```python
from build123d import *

# Parameters (mm, degrees)
SKETCH1_W                        = 63.5
SKETCH1_H                        = 25.4
BOSS_EXTRUDE1_DEPTH              = 20.32
F_10_0_1935_DIAMETER_HOLE1_D     = 4.9149
F_10_0_1935_DIAMETER_HOLE1_DEPTH = 15.875
F_10_0_1935_DIAMETER_HOLE1_TIP   = 1.476584928
F_10_0_1935_DIAMETER_HOLE2_D     = 4.9149
F_10_0_1935_DIAMETER_HOLE2_DEPTH = 10.16
F_10_0_1935_DIAMETER_HOLE2_TIP   = 1.476584928
SKETCH6_R                        = 3.175
CUT_EXTRUDE1_DEPTH               = 59.427173695
SKETCH7_R                        = 7.62
CUT_EXTRUDE2_DEPTH               = 7.62
TAP_DRILL_FOR_M6X1_0_TAP1_D      = 5
TAP_DRILL_FOR_M6X1_0_TAP1_DEPTH  = 16.002
TAP_DRILL_FOR_M6X1_0_TAP1_TIP    = 1.502151548


with BuildPart() as part:
    # Sketch1 → Boss-Extrude1 (new body)
    with BuildSketch(Plane.XY):
        with Locations((-16.785267857, -8.961160714)):
            Rectangle(SKETCH1_W, SKETCH1_H)
    extrude(amount=BOSS_EXTRUDE1_DEPTH)

    # #10 (0.1935) Diameter Hole1
    with Locations(Plane(origin=(14.964732143, 0, 0), x_dir=(0, 0, -1), z_dir=(1, 0, 0))):
        with Locations((-10.16, -15.311160714)):
            Hole(F_10_0_1935_DIAMETER_HOLE1_D / 2, depth=F_10_0_1935_DIAMETER_HOLE1_DEPTH)
            with Locations((0, 0, -(F_10_0_1935_DIAMETER_HOLE1_DEPTH + F_10_0_1935_DIAMETER_HOLE1_TIP / 2))):  # 118° drill point
                Cone(0, F_10_0_1935_DIAMETER_HOLE1_D / 2, F_10_0_1935_DIAMETER_HOLE1_TIP, mode=Mode.SUBTRACT)

    # #10 (0.1935) Diameter Hole2
    with Locations(Plane.XY.offset(20.32)):
        with Locations((-0.910267857, -15.311160714)):
            Hole(F_10_0_1935_DIAMETER_HOLE2_D / 2, depth=F_10_0_1935_DIAMETER_HOLE2_DEPTH)
            with Locations((0, 0, -(F_10_0_1935_DIAMETER_HOLE2_DEPTH + F_10_0_1935_DIAMETER_HOLE2_TIP / 2))):  # 118° drill point
                Cone(0, F_10_0_1935_DIAMETER_HOLE2_D / 2, F_10_0_1935_DIAMETER_HOLE2_TIP, mode=Mode.SUBTRACT)

    # Sketch6 → Cut-Extrude1 (cut, through all)
    with BuildSketch(Plane(origin=(0, -21.661160714, 0), x_dir=(-1, 0, 0), z_dir=(0, -1, 0))):
        with Locations(Location((0.910267857, -10.16, 0), (0, 0, 90))):
            Circle(SKETCH6_R)
    extrude(amount=-CUT_EXTRUDE1_DEPTH, mode=Mode.SUBTRACT)

    # Sketch7 → Cut-Extrude2 (cut)
    with BuildSketch(Plane(origin=(0, 3.738839286, 0), x_dir=(1, 0, 0), z_dir=(0, 1, 0))):
        with Locations(Location((-0.910267857, -10.16, 0), (0, 0, 270))):
            Circle(SKETCH7_R)
    extrude(amount=-CUT_EXTRUDE2_DEPTH, mode=Mode.SUBTRACT)

    # Tap Drill for M6x1.0 Tap1
    with Locations(Plane(origin=(0, 3.738839286, 0), x_dir=(1, 0, 0), z_dir=(0, 1, 0))):
        with Locations((-43.455267857, -10.16)):
            Hole(TAP_DRILL_FOR_M6X1_0_TAP1_D / 2, depth=TAP_DRILL_FOR_M6X1_0_TAP1_DEPTH)
            with Locations((0, 0, -(TAP_DRILL_FOR_M6X1_0_TAP1_DEPTH + TAP_DRILL_FOR_M6X1_0_TAP1_TIP / 2))):  # 118° drill point
                Cone(0, TAP_DRILL_FOR_M6X1_0_TAP1_D / 2, TAP_DRILL_FOR_M6X1_0_TAP1_TIP, mode=Mode.SUBTRACT)


solid = part.part
```
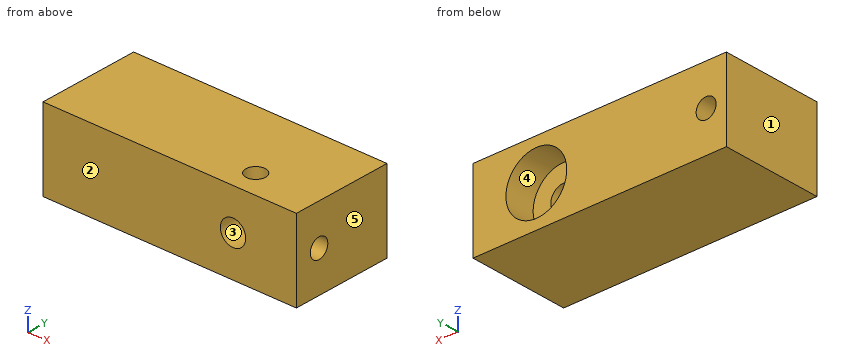
Check sheet for the modelled part. Datum: model origin and axes. Units: mm. Face numbers are marked on the shaded views. A direction names the side the tool comes from. Coordinates: 2 decimals unless noted, no trailing zeros. Loops run counter-clockwise (first coordinate to the right, second up) from the corner with the lowest first, then second, coordinate; pieces in that order, holes last.
1) Sectioned sample at C-C (y = -9). Record the boundary of the cut face in (x, z) (3 decimals).
2) Material ranges on probe 1 along X at (y, z) = (-9.25, 10); probe 2 along Y at (x, z) = (5, 10.25); probe 3 along X at (y, z) = (-6, 8.75) (3 decimals), recorded low to high.
3) Gauge pin test, flat ends, axial feed: pin 1 (4 mm diameter, centred on x = -0.91, y = -15.31, fed in from +Z); pin 2 (7.5 mm diameter, centred on x = -0.91, z = 10.16, fed in from +Y). Record the tip position at first contact, or that the pin passes through.
4) Release check for a two-part mould opening along X. For the marked faces 1, 2 and 3 record: released by +X, released by -X, zero draft, split by the parting line, or undercut.
5) Sectioned sample at D-D (y = 0.25). Record the boundary of the cut face in (x, z).
6) Sectioned sample at A-A (z = 16.25). Record the boundary of the cut face in (x, y).
7) Sectioned sample at B-B (x = 4). Record the boundary of the cut face in (y, z), and give its area (3 significant figures).
8) Access from +Z, -Z, +X, -X, +Y, -Y to the whole of each face (thin tool, end or side, straight path). Record for the marked faces 4 and 5.
Check sheet entries:
1. outline: (-48.535, 0) - (14.965, 0) - (14.965, 20.32) - (-48.535, 20.32) - close; hole circle Ø5 at (-43.455, 10.16); hole circle Ø6.35 at (-0.91, 10.16)
2. probe 1: x = -48.54 to -45.95, -40.96 to -4.08, 2.26 to 14.96
2. probe 2: y = -21.66 to -17.77, -12.86 to -3.88
2. probe 3: x = -48.535 to -45.52, -41.391 to -3.755, 1.934 to 14.965
3. pin 1: stops at z = 7.69
3. pin 2: stops at y = -3.88
4. face 1: released by -X
4. face 2: zero draft
4. face 3: undercut
5. outline: (-48.54, 0) - (14.96, 0) - (14.96, 20.32) - (-48.54, 20.32) - close; hole circle Ø5 at (-43.46, 10.16); hole circle Ø15.24 at (-0.91, 10.16)
6. outline: (-48.54, -21.66) - (14.96, -21.66) - (14.96, 3.74) - (3.67, 3.74) - (3.67, -3.88) - (-5.49, -3.88) - (-5.49, 3.74) - (-48.54, 3.74) - close; hole circle Ø4.91 at (-0.91, -15.31)
7. outline: (-21.66, 0) - (3.74, 0) - (3.74, 4.33) - (-3.88, 4.33) - (-3.88, 15.99) - (3.74, 15.99) - (3.74, 20.32) - (-21.66, 20.32) - close; hole circle Ø4.91 at (-15.31, 10.16)
7. area: 408 mm2
8. face 4: +Y
8. face 5: +Z, -Z, +X, +Y, -Y
